```python
from build123d import *

# Parameters (mm, degrees)
SKETCH_2_W          = 6
SKETCH_2_H          = 0.5
EXTRUDE_1_DEPTH     = 6
SKETCH_3_R          = 1.65
CUT_EXTRUDE_1_DEPTH = 3.5
FILLET_1_R          = 0.5
FILLET_2_R          = 2


with BuildPart() as part:
    # Эскиз1 → Повернуть1 (revolve)
    with BuildSketch(Plane.XY, mode=Mode.PRIVATE) as revolve_1_sk:
        Polygon((0, 0), (0, 93.5), (2.5, 93.5), (2.5, 82.5), (8.75, 82.5), (8.75, 78), (21.25, 78), (21.25, 73), (22.5, 73), (22.5, 35), (21.25, 35), (21.25, 11.5), (8.75, 11.5), (8.75, 7.5), (2.5, 7.5), (2.5, 0), align=None)
    revolve(revolve_1_sk.sketch.rotate(Axis((0, 0, 0), (0, 1, 0)), 90), axis=Axis((0, 0, 0), (0, 1, 0)))

    # Эскиз2 → Бобышка-Вытянуть1 (add)
    with BuildSketch(Plane.XZ.offset(-11.5)):
        with Locations((0, -19)):
            Rectangle(SKETCH_2_W, SKETCH_2_H)
        with Locations((0, 19)):
            Rectangle(SKETCH_2_W, SKETCH_2_H)
    extrude(amount=EXTRUDE_1_DEPTH)

    # Эскиз3 → Вырез-Вытянуть1 (cut)
    with BuildSketch(Plane(origin=(0, 78, 0), x_dir=(1, 0, 0), z_dir=(0, 1, 0))):
        with Locations(Location((0, -14.5, 0), (0, 0, 270))):
            Circle(SKETCH_3_R)
        with Locations(Location((0, 14.5, 0), (0, 0, 270))):
            Circle(SKETCH_3_R)
    extrude(amount=-CUT_EXTRUDE_1_DEPTH, mode=Mode.SUBTRACT)

    # Скругление1
    fillet_1_edges = [part.edges().sort_by_distance(p)[0] for p in [
        (0, 0, 2.5),
        (0, 7.5, 8.75),
        (0, 78, 21.25),
        (0, 82.5, 8.75),
        (0, 93.5, 2.5),
    ]]
    fillet(fillet_1_edges, radius=FILLET_1_R)

    # Скругление2
    fillet_2_edges = [part.edges().sort_by_distance(p)[0] for p in [
        (-3, 5.5, 19),
        (3, 5.5, 19),
        (-3, 5.5, -19),
        (3, 5.5, -19),
    ]]
    fillet(fillet_2_edges, radius=FILLET_2_R)


solid = part.part
```
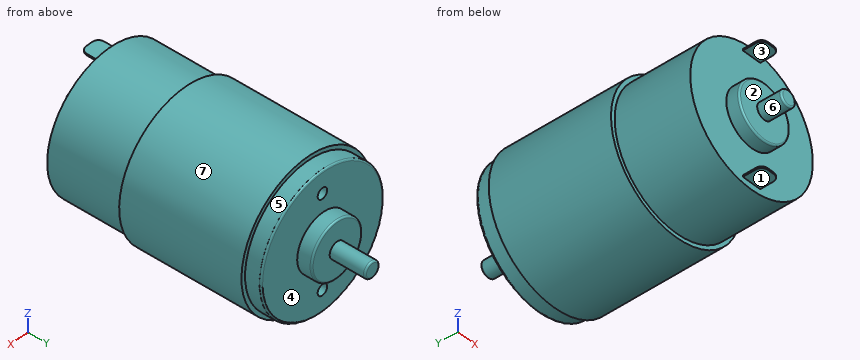
Geometry check sheet. Reference: the model listing, model coordinates, mm. Face numbers are marked on the shaded views. A direction names the side the tool comes from. Give positions to 0.01 mm unless a question says otherwise; leave off trailing zeros. Order: outer loops, then holes, each group sorted by start corner. A loop starts at its lowest first (then second) coordinate and runs counter-clockwise, first axis right, second up. Notation, with made-up numbers: (84.25, 12) -> (123.25, 12) arc R24 cw to (123.25, 27) -> close; hole circle Ø3 at (35.5, 26.5). An arc over 180 degrees is marked (long way). Write each question's results on one line, items separated by ' | '. Start each with the question number.
(1) Scan lines: line 1 (Y direction, x = -4, z = 2.5); line 2 (Y direction, x = -20, z = 0.5); line 3 (X direction, y = 76.95, z = -14.5). Record each from-to range of solid material in increasing order.
(2) Sectioned sample at A-A (y = 36.5). Enter the section's corners in (x, z), plus the area to 3 significant figures.
(3) Gauge pin test, flat ends, axial feed: P1, Ø12, axis at x = -14.5, y = 37, coming from the +Z side; P2, Ø3, axis at x = -1.5, y = 7.5, coming from the +Z side; P3, Ø0.6, axis at x = 0, z = 19, coming from the -Y side. Record the tip position at first contact, or that the pin passes through.
(4) Mould release check, pull along Z, two halves, no side actions. Record for the marked faces 1, 2, 3 and 4: pulls with the +Z half, pulls with the -Z half, needs draft (parallel to the pull), parting line crosses it, or undercut.
(5) Access from +Z, -Z, +X, -X, +Y, -Y to the whole of each face (thin tool, end or side, straight path). Record for the marked faces 5, 6 and 7.
(6) Sectioned sample at B-B (y = 84.5). Enter the section's corners in (x, z), plus the area to 3 significant figures.
Answer below:
1) line 1: 7.5 to 82.5 | line 2: 11.5 to 78 | line 3: -15.53 to -1.65, 1.65 to 15.53
2) outline: circle Ø45 at (0, 0) | area: 1,590 mm2
3) P1: z = 20.83 | P2: z = 19.25 | P3: y = 5.5
4) face 1: pulls with the -Z half | face 2: undercut | face 3: undercut | face 4: needs draft
5) face 5: +Y | face 6: -Y | face 7: +Y, -Y
6) outline: circle Ø5 at (0, 0) | area: 19.6 mm2
